For this review, take the finished solid that the model builds, in its own axes (mm). A direction names the side the tool comes from. Round coordinates to 2 decimals unless told otherwise and drop trailing zeros. Loops run counter-clockwise (first coordinate to the right, second up) from the corner with the lowest first, then second, coordinate; pieces in that order, holes last.
1) Take a section at B-B (z = 3). State the section outline as (x, y) points.
2) Tool access review of faces 5 (the flat face through (14, 7, -9.3)), 6 (the flat face through (14, 7, 9.3)), 7 (the flat face through (14, 7, 1.3)), 8 (the flat face through (14, 4.8, -7)), 9 (the flat face through (0, 4, 10.3)): name each direction out of +Z, -Z, +X, -X, +Y, -Y from which nothing blocks a thin tool from reaching the whole face with its end or side.
3) Mouldability with a two-part tool opening along Z and no side actions: class faces 1 (the flat face through (13.1, 3, 0)), 2 (the flat face through (0, 8.3, 0)), 3 (the cylindrical face through (-15.56, 4.52, 5.93)), 4 (the flat face through (14, 7, -5.1)) as pulls with the +Z half, pulls with the -Z half, needs draft (parallel to the pull), parting line crosses it, or undercut.
4) Wall thickness on L1, parallel to X at y = 6, z = 2.5; L2, parallel to X at y = 2, z = 4.25; L3, parallel to Y at x = -13.5, z = 5.5: over which ranges is each line inside the solid? List them lowest first.
5) Insertion check: pin 1 (1 mm diameter, centred on x = 13.5, y = 6, fed in from -Z); pin 2 (4 mm diameter, centred on y = 3.5, z = 2, fed in from -X); pin 3 (4 mm diameter, centred on y = 2.5, z = 0, fed in from +X); pin 4 (0.6 mm diameter, centred on x = 13.5, z = 5, fed in from -Y). Each pin has a flat end and moves straight along its axis. Give the tip position at first contact, or say it passes through.
6) Take a section at C-C (z = 5.25). State the section outline as (x, y) points, then the cut area to 3 significant figures.
7) Take a section at D-D (z = 0.75). State the section outline as (x, y) points.
8) Take a section at A-A (y = 6.75). State the section outline as (x, z) points, then the cut area to 3 significant figures.
```python
from build123d import *

# Parameters (mm, degrees)
SKETCH1_W           = 26.2
SKETCH1_H           = 20.6
BOSS_EXTRUDE1_DEPTH = 8.3
SKETCH2_W           = 8
SKETCH2_H           = 3.5
SKETCH2_W_2         = 4.2
BOSS_EXTRUDE2_DEPTH = 1.2
SKETCH3_R           = 0.95
BOSS_EXTRUDE3_DEPTH = 5


with BuildPart() as part:
    # Sketch1 → Boss-Extrude1 (new body)
    with BuildSketch(Plane(origin=(0, 0, 0), x_dir=(1, 0, 0), z_dir=(0, 1, 0))):
        Rectangle(SKETCH1_W, SKETCH1_H)
    extrude(amount=BOSS_EXTRUDE1_DEPTH)

    # Sketch2 → Boss-Extrude2 (add)
    with BuildSketch(Plane(origin=(13.1, 0, 0), x_dir=(0, 0, -1), z_dir=(1, 0, 0))):
        with Locations((-5.3, 6.55)):
            Rectangle(SKETCH2_W, SKETCH2_H)
        with Locations((7.2, 6.55)):
            Rectangle(SKETCH2_W_2, SKETCH2_H)
    extrude(amount=BOSS_EXTRUDE2_DEPTH)

    # Sketch3 → Boss-Extrude3 (add)
    with BuildSketch(Plane.ZY.offset(13.1)):
        with Locations(Location((5.174837269, 3.945319614, 0), (0, 0, 180))):
            Circle(SKETCH3_R)
    extrude(amount=BOSS_EXTRUDE3_DEPTH)


solid = part.part
```
Response:
1. outline: (-13.1, 0) - (13.1, 0) - (13.1, 4.8) - (14.3, 4.8) - (14.3, 8.3) - (-13.1, 8.3) - close
2. face 5: -Z, +X, +Y, -Y
2. face 6: +Z, +X, +Y, -Y
2. face 7: +X, +Y, -Y
2. face 8: +Z, -Z, +X, -Y
2. face 9: +Z, +X, -X, +Y, -Y
3. face 1: undercut
3. face 2: needs draft
3. face 3: parting line crosses it
3. face 4: undercut
4. L1: x = -13.1 to 14.3
4. L2: x = -13.1 to 13.1
4. L3: y = 3.05 to 4.84
5. pin 1: stops at z = -10.3
5. pin 2: stops at x = -13.1
5. pin 3: stops at x = 13.1
5. pin 4: stops at y = 4.8
6. outline: (-18.1, 3) - (-13.1, 3) - (-13.1, 0) - (13.1, 0) - (13.1, 4.8) - (14.3, 4.8) - (14.3, 8.3) - (-13.1, 8.3) - (-13.1, 4.89) - (-18.1, 4.89) - close
6. area: 231 mm2
7. outline: (-13.1, 0) - (13.1, 0) - (13.1, 8.3) - (-13.1, 8.3) - close
8. outline: (-13.1, -10.3) - (13.1, -10.3) - (13.1, -9.3) - (14.3, -9.3) - (14.3, -5.1) - (13.1, -5.1) - (13.1, 1.3) - (14.3, 1.3) - (14.3, 9.3) - (13.1, 9.3) - (13.1, 10.3) - (-13.1, 10.3) - close
8. area: 554 mm2
